Build history of the part. All positions in model axes, mm. A direction names the side the tool comes from. Round coordinates to 2 decimals unless told otherwise and drop trailing zeros. Loops run counter-clockwise (first coordinate to the right, second up) from the corner with the lowest first, then second, coordinate; pieces in that order, holes last. Notation, with made-up numbers: M -34,-21.5 L 11,-21.5 A25 cw 11,17.5 Z; hole C 37.5,63.25 d6. An arc over 180 degrees is marked long. One line per item, written item: value.
```python
from build123d import *

# Parameters (mm, degrees)
F1_R     = 1.75
F2_DEPTH = 3


with BuildPart() as f2:
    # F1 (on Right) → F2 (new body)
    with BuildSketch(Plane.YZ):
        with BuildLine():
            Line((-50, 8), (-50, 0))
            Line((-50, 0), (-46.75, 0))
            Line((-46.75, 0), (-46.75, 2))
            Line((-46.75, 2), (-47.75, 2))
            Line((-47.75, 2), (-47.75, 6))
            Line((-47.75, 6), (-42.25, 6))
            Line((-42.25, 6), (-42.25, 2))
            Line((-42.25, 2), (-43.25, 2))
            Line((-43.25, 2), (-43.25, 0))
            Line((-43.25, 0), (-40, 0))
            Line((-40, 0), (-40, -5))
            Line((-40, -5), (-35, -5))
            Line((-35, -5), (-35, 0))
            Line((-35, 0), (-40, 6))
            ThreePointArc((-40, 6), (-33.354443, 20.434949), (-18.066553, 24.772184))
            Line((-18.066553, 24.772184), (29.429899, 17.350121))
            ThreePointArc((29.429899, 17.350121), (36.996677, 13.127923), (40, 5))
            Line((40, 5), (35, 0))
            Line((35, 0), (35, -5))
            Line((35, -5), (40, -5))
            Line((40, -5), (40, 0))
            Line((40, 0), (43.25, 0))
            Line((43.25, 0), (43.25, 1))
            Line((43.25, 1), (42.25, 1))
            Line((42.25, 1), (42.25, 5))
            Line((42.25, 5), (47.75, 5))
            Line((47.75, 5), (47.75, 1))
            Line((47.75, 1), (46.75, 1))
            Line((46.75, 1), (46.75, 0))
            Line((46.75, 0), (50, 0))
            Line((50, 0), (50, 6))
            ThreePointArc((50, 6), (46.217774, 16.330828), (36.659249, 21.777465))
            Line((36.659249, 21.777465), (-22.011127, 31.666197))
            ThreePointArc((-22.011127, 31.666197), (-41.496242, 26.32666), (-50, 8))
        make_face()
        with Locations((-45, 10)):
            Circle(F1_R, mode=Mode.SUBTRACT)
        with Locations((45, 9)):
            Circle(F1_R, mode=Mode.SUBTRACT)
        with Locations((-18.066553, 27.772184)):
            Circle(F1_R, mode=Mode.SUBTRACT)
        with Locations((29.429899, 20.350121)):
            Circle(F1_R, mode=Mode.SUBTRACT)
    extrude(amount=F2_DEPTH)


solid = f2.part
```
Item 1: Slice it at B-B, the plane y = -45. Give the cut face in (x, z), and give its area (3 significant figures).
Check values:
outline: M 0,6 L 3,6 L 3,8.25 L 0,8.25 Z; M 0,11.75 L 3,11.75 L 3,22.66 L 0,22.66 Z
area: 39.5 mm2
Item 2: Slice it at C-C, the plane x = 2.1. Give the number of separate pieces and of enclosed holes in the cut face, and give its area (3 significant figures).
Check values:
separate pieces: 1
enclosed holes: 4
area: 940 mm2
Item 3: Slice it at D-D, the plane y = -4. Give the cut face in (x, z).
Check values:
outline: M 0,22.57 L 3,22.57 L 3,28.63 L 0,28.63 Z
Item 4: Which spindle directions (+Z, -Z, +X, -X, +Y, -Y) get a long thin tool onto all of the face, cutting with end or side? Do faces 1 (the face through (1, -45, 6)), 2 (the face through (1, -48, 0)), 3 (the face through (1, -35, -3)). Say none if no direction does.
Check values:
face 1: +X, -X
face 2: -Z, +X, -X, -Y
face 3: -Z, +X, -X
Item 5: Drop flat-ended pins along their axis: P1, Ø1.5, axis at x = 1, y = -48, coming from the -Z side; P2, Ø1, axis at x = 1, y = 37.5, coming from the +Z side; P3, Ø2, axis at y = 45, z = 9, coming from the +X side; P4, Ø0.5, axis at x = 1, y = -43, coming from the +Z side. Give the stop position or say it passes through.
Check values:
P1: stops at z = 0
P2: stops at z = 21.72
P3: passes through
P4: stops at z = 25.19
Item 6: Pull direction Y, two halves, no side cores. Call faces 4 (the face through (1, 48, 0)), 5 (the face through (1, -50, 4)), 6 (the face through (1.479, -33.528, 20.285)): pulls with the +Y half, pulls with the -Y half, needs draft (parallel to the pull), parting line crosses it, or undercut.
Check values:
face 4: needs draft
face 5: pulls with the -Y half
face 6: undercut
Item 7: Wall check: line 1 along Y through (x, z) = (2.8, 3); line 2 along Z through (x, y) = (0.5, 43); line 3 along Z through (x, y) = (0.7, -45). Give the ranges that are in metal, low to high.
Check values:
line 1: y = -50 to -47.75, -42.25 to -37.5, 38 to 42.25, 47.75 to 50
line 2: z = 0 to 1, 5 to 19.23
line 3: z = 6 to 8.25, 11.75 to 22.66
Item 8: Slice it at A-A, the plane z = 4. Give the cut face in (x, y), and give its area (3 significant figures).
Check values:
outline: M 0,-50 L 3,-50 L 3,-47.75 L 0,-47.75 Z; M 0,-42.25 L 3,-42.25 L 3,-38.33 L 0,-38.33 Z; M 0,39 L 3,39 L 3,42.25 L 0,42.25 Z; M 0,47.75 L 3,47.75 L 3,50 L 0,50 Z
area: 35.0 mm2
